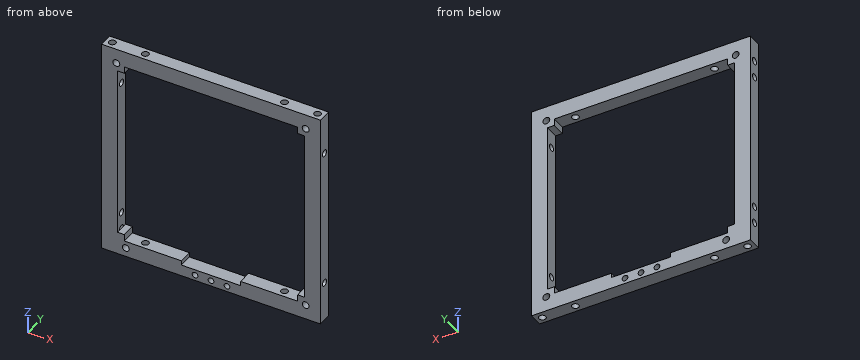
```python
from build123d import *

# Parameters (mm, degrees)
SKETCH1_W                       = 96
SKETCH1_H                       = 96
SKETCH1_W_2                     = 80
SKETCH1_H_2                     = 80
BOSS_EXTRUDE1_DEPTH             = 8
F_3_0_3_DIAMETER_HOLE6_D        = 3
F_3_0_3_DIAMETER_HOLE6_DEPTH    = 6
F_3_0_3_DIAMETER_HOLE3_D        = 3
F_3_0_3_DIAMETER_HOLE3_DEPTH    = 6
SKETCH27_W                      = 82
SKETCH27_H                      = 82
CUT_EXTRUDE2_DEPTH              = 10
F_3_0_3_DIAMETER_HOLE1_D        = 3
F_3_0_3_DIAMETER_HOLE2_D        = 3
SKETCH35_W                      = 3
SKETCH35_H                      = 3
BOSS_EXTRUDE2_DEPTH             = 8
F_3_0_3_DIAMETER_HOLE7_D        = 3
SKETCH44_W                      = 96
SKETCH44_H                      = 1
CUT_EXTRUDE4_DEPTH              = 142
SKETCH47_W                      = 14
SKETCH47_H                      = 2
CUT_EXTRUDE5_DEPTH              = 10
F_2_5_2_5_DIAMETER_HOLE1_D      = 2.5
TAP_DRILL_FOR_M3X0_5_TAP3_D     = 3
TAP_DRILL_FOR_M3X0_5_TAP3_DEPTH = 7
SKETCH54_W                      = 6
SKETCH54_H                      = 6
CUT_EXTRUDE6_DEPTH              = 2


with BuildPart() as part:
    # Sketch1 → Boss-Extrude1 (new body)
    with BuildSketch(Plane(origin=(0, 0, 0), x_dir=(1, 0, 0), z_dir=(0, 1, 0))):
        Rectangle(SKETCH1_W, SKETCH1_H)
        Rectangle(SKETCH1_W_2, SKETCH1_H_2, mode=Mode.SUBTRACT)
    extrude(amount=BOSS_EXTRUDE1_DEPTH)

    # Ø3.0 (3) Diameter Hole6
    with Locations(Plane.XY.offset(48)):
        with Locations((45, 4), (-45, 4)):
            Hole(F_3_0_3_DIAMETER_HOLE6_D / 2, depth=F_3_0_3_DIAMETER_HOLE6_DEPTH)

    # Ø3.0 (3) Diameter Hole3
    with Locations(Plane(origin=(0, 0, -48), x_dir=(-1, 0, 0), z_dir=(0, 0, -1))):
        with Locations((-45, 4), (45, 4)):
            Hole(F_3_0_3_DIAMETER_HOLE3_D / 2, depth=F_3_0_3_DIAMETER_HOLE3_DEPTH)

    # Sketch27 → Cut-Extrude2 (cut)
    with BuildSketch(Plane(origin=(0, 8, 0), x_dir=(1, 0, 0), z_dir=(0, 1, 0))):
        Rectangle(SKETCH27_W, SKETCH27_H)
    extrude(amount=-CUT_EXTRUDE2_DEPTH, mode=Mode.SUBTRACT)

    # Ø3.0 (3) Diameter Hole1 (through all)
    with Locations(Plane.XY.offset(48)):
        with Locations((-30.5, 4), (30.5, 4)):
            Hole(F_3_0_3_DIAMETER_HOLE1_D / 2)

    # Ø3.0 (3) Diameter Hole2 (through all)
    with Locations(Plane.ZY.offset(48)):
        with Locations((-30.5, 4), (30.5, 4)):
            Hole(F_3_0_3_DIAMETER_HOLE2_D / 2)

    # Sketch35 → Boss-Extrude2 (add)
    with BuildSketch(Plane(origin=(0, 8, 0), x_dir=(1, 0, 0), z_dir=(0, 1, 0))):
        with Locations((39.5, -39.5)):
            Rectangle(SKETCH35_W, SKETCH35_H)
        with Locations((-39.5, 39.5)):
            Rectangle(SKETCH35_W, SKETCH35_H)
        with Locations((39.5, 39.5)):
            Rectangle(SKETCH35_W, SKETCH35_H)
        with Locations((-39.5, -39.5)):
            Rectangle(SKETCH35_W, SKETCH35_H)
    extrude(amount=-BOSS_EXTRUDE2_DEPTH)

    # Ø3.0 (3) Diameter Hole7 (through all)
    with Locations(Plane(origin=(0, 8, 0), x_dir=(1, 0, 0), z_dir=(0, 1, 0))):
        with Locations((-37.33, 44.05), (41.5, 41.5), (41.5, -41.5), (-41.5, -41.5)):
            Hole(F_3_0_3_DIAMETER_HOLE7_D / 2)

    # Sketch44 → Cut-Extrude4 (cut)
    with BuildSketch(Plane(origin=(0, 0, -48), x_dir=(-1, 0, 0), z_dir=(0, 0, -1))):
        with Locations((0, 7.5)):
            Rectangle(SKETCH44_W, SKETCH44_H)
        with Locations((0, 0.5)):
            Rectangle(SKETCH44_W, SKETCH44_H)
    extrude(amount=-CUT_EXTRUDE4_DEPTH, mode=Mode.SUBTRACT)

    # Sketch47 → Cut-Extrude5 (cut)
    with BuildSketch(Plane(origin=(0, 7, 0), x_dir=(1, 0, 0), z_dir=(0, 1, 0))):
        with Locations((0, 42)):
            Rectangle(SKETCH47_W, SKETCH47_H)
    extrude(amount=-CUT_EXTRUDE5_DEPTH, mode=Mode.SUBTRACT)

    # Ø2.5 (2.5) Diameter Hole1 (through all)
    with Locations(Plane(origin=(0, 1, 0), x_dir=(-1, 0, 0), z_dir=(0, -1, 0))):
        with Locations((7, 45.5), (0, 45.5), (-7, 45.5)):
            Hole(F_2_5_2_5_DIAMETER_HOLE1_D / 2)

    # Tap Drill for M3x0.5 Tap3
    with Locations(Plane.ZY.offset(48)):
        with Locations((38.1, 4), (-38.1, 4)):
            Hole(TAP_DRILL_FOR_M3X0_5_TAP3_D / 2, depth=TAP_DRILL_FOR_M3X0_5_TAP3_DEPTH)

    # Sketch54 → Cut-Extrude6 (cut)
    with BuildSketch(Plane.XY.offset(-41)):
        with Locations((-10, 4)):
            Rectangle(SKETCH54_W, SKETCH54_H)
        with Locations((10, 4)):
            Rectangle(SKETCH54_W, SKETCH54_H)
    extrude(amount=-CUT_EXTRUDE6_DEPTH, mode=Mode.SUBTRACT)


solid = part.part
```
CAD build for the part. Positions are in the model's coordinates, mm. Coordinates: 2 decimals unless noted, no trailing zeros. Loops run counter-clockwise (first coordinate to the right, second up) from the corner with the lowest first, then second, coordinate; pieces in that order, holes last. Notation, with made-up numbers: (29.25, -10.75) - (45.25, -10.75) arc R24 ccw to (45.25, 13.25) - close; hole circle Ø8 at (5.25, 38). An arc over 180 degrees is marked (long way). Use CSV: the item, a comma, the result in double quotes. Start each with the question number.
Q1. Cut at C-C, the plane x = -7. List the corners of the cut face in (y, z).
Q2. Cut at D-D, the plane x = 45. List the corners of the cut face in (y, z), then the cut area to 3 significant figures.
Q3. Cut at B-B, the plane z = -1. List the corners of the cut face in (x, y).
Q4. Drop flat-ended pins along their axis: P1, Ø2.5, axis at x = -30.5, y = 4, coming from the +Z side; P2, Ø2.5, axis at x = -45, y = 4, coming from the +Z side; P3, Ø0.5, axis at y = 4.5, z = -39, coming from the -X side; P4, Ø2.5, axis at x = -45, y = 4, coming from the -Z side. Give the stop position or say it passes through.
Q5. Probe probe 1 along X at (y, z) = (2.2, 30.5); probe 2 along Z at (x, y) = (5, 2.7). List the from-to ranges inside material, lowest first. Write a range as from..to.
Q6. Cut at A-A, the plane x = -18. List the corners of the cut face in (y, z), then the cut area to 3 significant figures.
Here are the results:
1,outline,"(1, -48) - (7, -48) - (7, -46.75) - (1, -46.75) - close; (1, -44.25) - (7, -44.25) - (7, -43) - (1, -43) - close; (1, 41) - (7, 41) - (7, 48) - (1, 48) - close"
2,outline,"(1, -48) - (2.5, -48) - (2.5, -42) - (5.5, -42) - (5.5, -48) - (7, -48) - (7, 48) - (5.5, 48) - (5.5, 42) - (2.5, 42) - (2.5, 48) - (1, 48) - close; hole circle Ø3 at (4, -30.5); hole circle Ø3 at (4, 30.5)"
2,area,"526 mm2"
3,outline,"(-48, 1) - (-41, 1) - (-41, 7) - (-48, 7) - close; (41, 1) - (48, 1) - (48, 7) - (41, 7) - close"
4,P1,"through"
4,P2,"z = 42"
4,P3,"x = -41"
4,P4,"z = -42"
5,probe 1,"-48..-41, 41..48"
5,probe 2,"-48..-43, 41..48"
6,outline,"(1, -48) - (7, -48) - (7, -41) - (1, -41) - close; (1, 41) - (7, 41) - (7, 48) - (1, 48) - close"
6,area,"84.0 mm2"
